Could you check a few things on this model? Use its own coordinates, in mm. A direction names the side the tool comes from. Give positions to 0.01 mm unless a question says otherwise; leave off trailing zeros. Order: outer loops, then holes, each group sorted by start corner. A loop starts at its lowest first (then second) coordinate and runs counter-clockwise, first axis right, second up. Notation, with made-up numbers: M -26.5,11 L 6.5,11 A24 cw 6.5,47 Z; hole C 74,65 d6. An arc over 180 degrees is marked long. Return JSON: item names as keys, results as strings. Group by question number.
```python
from build123d import *

# Parameters (mm, degrees)
BOSS_EXTRUDE1_DEPTH = 6.35


with BuildPart() as part:
    # Sketch1 → Boss-Extrude1 (new body)
    with BuildSketch(Plane(origin=(0, 0, 0), x_dir=(1, 0, 0), z_dir=(0, 1, 0))):
        with BuildLine():
            Line((-147.307889143, -110), (147.307889143, -110))
            ThreePointArc((147.307889143, -110), (158.024259459, -106.886663592), (165.404263187, -98.515940727))
            Line((165.404263187, -98.515940727), (218.096374044, 13.454794844))
            ThreePointArc((218.096374044, 13.454794844), (219.518292457, 17.607679352), (220, 21.97073557))
            Line((220, 21.97073557), (220, 140))
            ThreePointArc((220, 140), (214.142135624, 154.142135624), (200, 160))
            Line((200, 160), (-200, 160))
            ThreePointArc((-200, 160), (-214.142135624, 154.142135624), (-220, 140))
            Line((-220, 140), (-220, 21.97073557))
            ThreePointArc((-220, 21.97073557), (-219.518292457, 17.607679352), (-218.096374044, 13.454794844))
            Line((-218.096374044, 13.454794844), (-165.404263187, -98.515940727))
            ThreePointArc((-165.404263187, -98.515940727), (-158.024259459, -106.886663592), (-147.307889143, -110))
        make_face()
        with BuildLine():
            Line((-170, 127.5), (-170, 27.5))
            ThreePointArc((-170, 27.5), (-187.5, 10), (-205, 27.5))
            Line((-205, 27.5), (-205, 127.5))
            ThreePointArc((-205, 127.5), (-187.5, 145), (-170, 127.5))
        make_face(mode=Mode.SUBTRACT)
        with BuildLine():
            Line((-132.5, 145), (-32.5, 145))
            ThreePointArc((-32.5, 145), (-15, 127.5), (-32.5, 110))
            Line((-32.5, 110), (-132.5, 110))
            ThreePointArc((-132.5, 110), (-150, 127.5), (-132.5, 145))
        make_face(mode=Mode.SUBTRACT)
        with BuildLine():
            Line((205, 127.5), (205, 27.5))
            ThreePointArc((205, 27.5), (187.5, 10), (170, 27.5))
            Line((170, 27.5), (170, 127.5))
            ThreePointArc((170, 127.5), (187.5, 145), (205, 127.5))
        make_face(mode=Mode.SUBTRACT)
        with BuildLine():
            Line((32.5, 145), (132.5, 145))
            ThreePointArc((132.5, 145), (150, 127.5), (132.5, 110))
            Line((132.5, 110), (32.5, 110))
            ThreePointArc((32.5, 110), (15, 127.5), (32.5, 145))
        make_face(mode=Mode.SUBTRACT)
    extrude(amount=BOSS_EXTRUDE1_DEPTH)


solid = part.part
```
1. Imagine slicing it at D-D, the plane x = 187.5. Please give me the cut outline in (y, z).
2. I need wall thicknesses on L1, parallel to X at y = 5.75, z = -26.5; L2, parallel to Z at x = -133, y = 0.5; L3, parallel to X at y = 2.5, z = -142.5. Which ranges of each line are inside material? Lowest first, please. Write a range as from..to.
3. Imagine slicing it at A-A, the plane z = -86.5. Please give me the cut outline in (x, y), plus the area to 3 significant figures.
4. If we mould it in two halves opening along X, with no side actions, what happens to faces 3 (the cylindrical face through (-158.16, 3.13, 106.8)), 4 (the cylindrical face through (187.115, 3.131, -144.996)), 5 (the flat face through (-3, 6.35, -27))? For each: pulls with the +X half, pulls with the -X half, needs draft (parallel to the pull), parting line crosses it, or undercut.
5. Imagine slicing it at B-B, the plane y = 1.75. Please give me the cut outline in (x, z), plus the area to 3 significant figures.
6. Imagine slicing it at C-C, the plane x = -50. Please give me the cut outline in (y, z), plus the area to 3 significant figures.
7. Which directions (+Z, -Z, +X, -X, +Y, -Y) give clear straight access to the entire face, cutting with the end or side of a thin tool? Please do faces 1 (the cylindrical face through (-149.996, 3.131, -127.115)), 2 (the flat face through (191.381, 3.131, 43.314)).
Values:
{
 "1": {"outline": "M 0,-160 L 6.35,-160 L 6.35,-145 L 0,-145 Z; M 0,-10 L 6.35,-10 L 6.35,51.56 L 0,51.56 Z"},
 "2": {"L1": "x = -220..-204.97, -170.03..170.03, 204.97..220", "L2": "z = -160..-144.99, -110.01..110", "L3": "x = -219.84..-196.51, -178.49..-141.51, -23.49..23.49, 141.51..178.49, 196.51..219.84"},
 "3": {"outline": "M -220,0 L -205,0 L -205,6.35 L -220,6.35 Z; M -170,0 L 170,0 L 170,6.35 L -170,6.35 Z; M 205,0 L 220,0 L 220,6.35 L 205,6.35 Z", "area": "2,350 mm²"},
 "4": {"face 3": "pulls with the -X half", "face 4": "undercut", "face 5": "needs draft"},
 "5": {"outline": "M -220,-140 A20 ccw -200,-160 L 200,-160 A20 ccw 220,-140 L 220,-21.97 A20 ccw 218.1,-13.45 L 165.4,98.52 A20 ccw 147.31,110 L -147.31,110 A20 ccw -165.4,98.52 L -218.1,-13.45 A20 ccw -220,-21.97 Z; hole M -205,-127.5 A17.5 ccw -170,-127.5 L -170,-27.5 A17.5 ccw -205,-27.5 Z; hole M -132.5,-145 L -32.5,-145 A17.5 ccw -32.5,-110 L -132.5,-110 A17.5 ccw Z; hole M 32.5,-145 L 132.5,-145 A17.5 ccw 132.5,-110 L 32.5,-110 A17.5 ccw Z; hole M 170,-127.5 A17.5 ccw 205,-127.5 L 205,-27.5 A17.5 ccw 170,-27.5 Z", "area": "93,100 mm²"},
 "6": {"outline": "M 0,-160 L 6.35,-160 L 6.35,-145 L 0,-145 Z; M 0,-110 L 6.35,-110 L 6.35,110 L 0,110 Z", "area": "1,490 mm²"},
 "7": {"face 1": "+Y, -Y", "face 2": "+Z, +X, +Y, -Y"}
}
